```python
from build123d import *

# Parameters (mm, degrees)
MODEL_R                 = 1.5
SALIENTE_EXTRUIR1_DEPTH = 3


with BuildPart() as part:
    # Model → Saliente-Extruir1 (new body)
    with BuildSketch(Plane.XY):
        with BuildLine():
            Line((256.429131311, 228.742243614), (364.429131311, 228.742243614))
            ThreePointArc((364.429131311, 228.742243614), (367.611111826, 227.424224129), (368.929131311, 224.242243614))
            Line((368.929131311, 224.242243614), (368.929131311, 215.242243614))
            ThreePointArc((368.929131311, 215.242243614), (367.611111826, 212.060263099), (364.429131311, 210.742243614))
            Line((364.429131311, 210.742243614), (256.429131311, 210.742243614))
            ThreePointArc((256.429131311, 210.742243614), (253.247150795, 212.060263099), (251.929131311, 215.242243614))
            Line((251.929131311, 215.242243614), (251.929131311, 224.242243614))
            ThreePointArc((251.929131311, 224.242243614), (253.247150795, 227.424224129), (256.429131311, 228.742243614))
        make_face()
        with Locations((337.429131311, 215.242243614)):
            Circle(MODEL_R, mode=Mode.SUBTRACT)
        with Locations((319.429131311, 215.242243614)):
            Circle(MODEL_R, mode=Mode.SUBTRACT)
        with Locations((328.429131311, 215.242243614)):
            Circle(MODEL_R, mode=Mode.SUBTRACT)
        with Locations((310.429131311, 215.242243614)):
            Circle(MODEL_R, mode=Mode.SUBTRACT)
        with Locations((292.429131311, 215.242243614)):
            Circle(MODEL_R, mode=Mode.SUBTRACT)
        with Locations((301.429131311, 215.242243614)):
            Circle(MODEL_R, mode=Mode.SUBTRACT)
        with Locations((274.429131311, 215.242243614)):
            Circle(MODEL_R, mode=Mode.SUBTRACT)
        with Locations((283.429131311, 215.242243614)):
            Circle(MODEL_R, mode=Mode.SUBTRACT)
        with Locations((265.429131311, 215.242243614)):
            Circle(MODEL_R, mode=Mode.SUBTRACT)
        with Locations((256.429131311, 215.242243614)):
            Circle(MODEL_R, mode=Mode.SUBTRACT)
        with Locations((346.429131311, 215.242243614)):
            Circle(MODEL_R, mode=Mode.SUBTRACT)
        with Locations((355.429131311, 215.242243614)):
            Circle(MODEL_R, mode=Mode.SUBTRACT)
        with Locations((364.429131311, 215.242243614)):
            Circle(MODEL_R, mode=Mode.SUBTRACT)
        with BuildLine():
            Line((267.929131311, 222.617243614), (262.929131311, 222.617243614))
            ThreePointArc((262.929131311, 222.617243614), (262.398801225, 222.836913528), (262.179131311, 223.367243614))
            Line((262.179131311, 223.367243614), (262.179131311, 225.117243614))
            ThreePointArc((262.179131311, 225.117243614), (262.398801225, 225.6475737), (262.929131311, 225.867243614))
            Line((262.929131311, 225.867243614), (267.929131311, 225.867243614))
            ThreePointArc((267.929131311, 225.867243614), (268.459461397, 225.6475737), (268.679131311, 225.117243614))
            Line((268.679131311, 225.117243614), (268.679131311, 223.367243614))
            ThreePointArc((268.679131311, 223.367243614), (268.459461397, 222.836913528), (267.929131311, 222.617243614))
        make_face(mode=Mode.SUBTRACT)
        with BuildLine():
            Line((285.929131311, 222.617243614), (280.929131311, 222.617243614))
            ThreePointArc((280.929131311, 222.617243614), (280.398801225, 222.836913528), (280.179131311, 223.367243614))
            Line((280.179131311, 223.367243614), (280.179131311, 225.117243614))
            ThreePointArc((280.179131311, 225.117243614), (280.398801225, 225.6475737), (280.929131311, 225.867243614))
            Line((280.929131311, 225.867243614), (285.929131311, 225.867243614))
            ThreePointArc((285.929131311, 225.867243614), (286.459461397, 225.6475737), (286.679131311, 225.117243614))
            Line((286.679131311, 225.117243614), (286.679131311, 223.367243614))
            ThreePointArc((286.679131311, 223.367243614), (286.459461397, 222.836913528), (285.929131311, 222.617243614))
        make_face(mode=Mode.SUBTRACT)
        with BuildLine():
            Line((258.929131311, 222.617243614), (253.929131311, 222.617243614))
            ThreePointArc((253.929131311, 222.617243614), (253.398801225, 222.836913528), (253.179131311, 223.367243614))
            Line((253.179131311, 223.367243614), (253.179131311, 225.117243614))
            ThreePointArc((253.179131311, 225.117243614), (253.398801225, 225.6475737), (253.929131311, 225.867243614))
            Line((253.929131311, 225.867243614), (258.929131311, 225.867243614))
            ThreePointArc((258.929131311, 225.867243614), (259.459461397, 225.6475737), (259.679131311, 225.117243614))
            Line((259.679131311, 225.117243614), (259.679131311, 223.367243614))
            ThreePointArc((259.679131311, 223.367243614), (259.459461397, 222.836913528), (258.929131311, 222.617243614))
        make_face(mode=Mode.SUBTRACT)
        with BuildLine():
            Line((276.929131311, 222.617243614), (271.929131311, 222.617243614))
            ThreePointArc((271.929131311, 222.617243614), (271.398801225, 222.836913528), (271.179131311, 223.367243614))
            Line((271.179131311, 223.367243614), (271.179131311, 225.117243614))
            ThreePointArc((271.179131311, 225.117243614), (271.398801225, 225.6475737), (271.929131311, 225.867243614))
            Line((271.929131311, 225.867243614), (276.929131311, 225.867243614))
            ThreePointArc((276.929131311, 225.867243614), (277.459461397, 225.6475737), (277.679131311, 225.117243614))
            Line((277.679131311, 225.117243614), (277.679131311, 223.367243614))
            ThreePointArc((277.679131311, 223.367243614), (277.459461397, 222.836913528), (276.929131311, 222.617243614))
        make_face(mode=Mode.SUBTRACT)
        with BuildLine():
            Line((294.929131311, 222.617243614), (289.929131311, 222.617243614))
            ThreePointArc((289.929131311, 222.617243614), (289.398801225, 222.836913528), (289.179131311, 223.367243614))
            Line((289.179131311, 223.367243614), (289.179131311, 225.117243614))
            ThreePointArc((289.179131311, 225.117243614), (289.398801225, 225.6475737), (289.929131311, 225.867243614))
            Line((289.929131311, 225.867243614), (294.929131311, 225.867243614))
            ThreePointArc((294.929131311, 225.867243614), (295.459461397, 225.6475737), (295.679131311, 225.117243614))
            Line((295.679131311, 225.117243614), (295.679131311, 223.367243614))
            ThreePointArc((295.679131311, 223.367243614), (295.459461397, 222.836913528), (294.929131311, 222.617243614))
        make_face(mode=Mode.SUBTRACT)
        with BuildLine():
            Line((303.929131311, 222.617243614), (298.929131311, 222.617243614))
            ThreePointArc((298.929131311, 222.617243614), (298.398801225, 222.836913528), (298.179131311, 223.367243614))
            Line((298.179131311, 223.367243614), (298.179131311, 225.117243614))
            ThreePointArc((298.179131311, 225.117243614), (298.398801225, 225.6475737), (298.929131311, 225.867243614))
            Line((298.929131311, 225.867243614), (303.929131311, 225.867243614))
            ThreePointArc((303.929131311, 225.867243614), (304.459461397, 225.6475737), (304.679131311, 225.117243614))
            Line((304.679131311, 225.117243614), (304.679131311, 223.367243614))
            ThreePointArc((304.679131311, 223.367243614), (304.459461397, 222.836913528), (303.929131311, 222.617243614))
        make_face(mode=Mode.SUBTRACT)
        with BuildLine():
            Line((321.929131311, 222.617243614), (316.929131311, 222.617243614))
            ThreePointArc((316.929131311, 222.617243614), (316.398801225, 222.836913528), (316.179131311, 223.367243614))
            Line((316.179131311, 223.367243614), (316.179131311, 225.117243614))
            ThreePointArc((316.179131311, 225.117243614), (316.398801225, 225.6475737), (316.929131311, 225.867243614))
            Line((316.929131311, 225.867243614), (321.929131311, 225.867243614))
            ThreePointArc((321.929131311, 225.867243614), (322.459461397, 225.6475737), (322.679131311, 225.117243614))
            Line((322.679131311, 225.117243614), (322.679131311, 223.367243614))
            ThreePointArc((322.679131311, 223.367243614), (322.459461397, 222.836913528), (321.929131311, 222.617243614))
        make_face(mode=Mode.SUBTRACT)
        with BuildLine():
            Line((312.929131311, 222.617243614), (307.929131311, 222.617243614))
            ThreePointArc((307.929131311, 222.617243614), (307.398801225, 222.836913528), (307.179131311, 223.367243614))
            Line((307.179131311, 223.367243614), (307.179131311, 225.117243614))
            ThreePointArc((307.179131311, 225.117243614), (307.398801225, 225.6475737), (307.929131311, 225.867243614))
            Line((307.929131311, 225.867243614), (312.929131311, 225.867243614))
            ThreePointArc((312.929131311, 225.867243614), (313.459461397, 225.6475737), (313.679131311, 225.117243614))
            Line((313.679131311, 225.117243614), (313.679131311, 223.367243614))
            ThreePointArc((313.679131311, 223.367243614), (313.459461397, 222.836913528), (312.929131311, 222.617243614))
        make_face(mode=Mode.SUBTRACT)
        with BuildLine():
            Line((357.929131311, 222.617243614), (352.929131311, 222.617243614))
            ThreePointArc((352.929131311, 222.617243614), (352.398801225, 222.836913528), (352.179131311, 223.367243614))
            Line((352.179131311, 223.367243614), (352.179131311, 225.117243614))
            ThreePointArc((352.179131311, 225.117243614), (352.398801225, 225.6475737), (352.929131311, 225.867243614))
            Line((352.929131311, 225.867243614), (357.929131311, 225.867243614))
            ThreePointArc((357.929131311, 225.867243614), (358.459461397, 225.6475737), (358.679131311, 225.117243614))
            Line((358.679131311, 225.117243614), (358.679131311, 223.367243614))
            ThreePointArc((358.679131311, 223.367243614), (358.459461397, 222.836913528), (357.929131311, 222.617243614))
        make_face(mode=Mode.SUBTRACT)
        with BuildLine():
            Line((348.929131311, 222.617243614), (343.929131311, 222.617243614))
            ThreePointArc((343.929131311, 222.617243614), (343.398801225, 222.836913528), (343.179131311, 223.367243614))
            Line((343.179131311, 223.367243614), (343.179131311, 225.117243614))
            ThreePointArc((343.179131311, 225.117243614), (343.398801225, 225.6475737), (343.929131311, 225.867243614))
            Line((343.929131311, 225.867243614), (348.929131311, 225.867243614))
            ThreePointArc((348.929131311, 225.867243614), (349.459461397, 225.6475737), (349.679131311, 225.117243614))
            Line((349.679131311, 225.117243614), (349.679131311, 223.367243614))
            ThreePointArc((349.679131311, 223.367243614), (349.459461397, 222.836913528), (348.929131311, 222.617243614))
        make_face(mode=Mode.SUBTRACT)
        with BuildLine():
            Line((339.929131311, 222.617243614), (334.929131311, 222.617243614))
            ThreePointArc((334.929131311, 222.617243614), (334.398801225, 222.836913528), (334.179131311, 223.367243614))
            Line((334.179131311, 223.367243614), (334.179131311, 225.117243614))
            ThreePointArc((334.179131311, 225.117243614), (334.398801225, 225.6475737), (334.929131311, 225.867243614))
            Line((334.929131311, 225.867243614), (339.929131311, 225.867243614))
            ThreePointArc((339.929131311, 225.867243614), (340.459461397, 225.6475737), (340.679131311, 225.117243614))
            Line((340.679131311, 225.117243614), (340.679131311, 223.367243614))
            ThreePointArc((340.679131311, 223.367243614), (340.459461397, 222.836913528), (339.929131311, 222.617243614))
        make_face(mode=Mode.SUBTRACT)
        with BuildLine():
            Line((330.929131311, 222.617243614), (325.929131311, 222.617243614))
            ThreePointArc((325.929131311, 222.617243614), (325.398801225, 222.836913528), (325.179131311, 223.367243614))
            Line((325.179131311, 223.367243614), (325.179131311, 225.117243614))
            ThreePointArc((325.179131311, 225.117243614), (325.398801225, 225.6475737), (325.929131311, 225.867243614))
            Line((325.929131311, 225.867243614), (330.929131311, 225.867243614))
            ThreePointArc((330.929131311, 225.867243614), (331.459461397, 225.6475737), (331.679131311, 225.117243614))
            Line((331.679131311, 225.117243614), (331.679131311, 223.367243614))
            ThreePointArc((331.679131311, 223.367243614), (331.459461397, 222.836913528), (330.929131311, 222.617243614))
        make_face(mode=Mode.SUBTRACT)
        with BuildLine():
            Line((366.929131311, 222.617243614), (361.929131311, 222.617243614))
            ThreePointArc((361.929131311, 222.617243614), (361.398801225, 222.836913528), (361.179131311, 223.367243614))
            Line((361.179131311, 223.367243614), (361.179131311, 225.117243614))
            ThreePointArc((361.179131311, 225.117243614), (361.398801225, 225.6475737), (361.929131311, 225.867243614))
            Line((361.929131311, 225.867243614), (366.929131311, 225.867243614))
            ThreePointArc((366.929131311, 225.867243614), (367.459461397, 225.6475737), (367.679131311, 225.117243614))
            Line((367.679131311, 225.117243614), (367.679131311, 223.367243614))
            ThreePointArc((367.679131311, 223.367243614), (367.459461397, 222.836913528), (366.929131311, 222.617243614))
        make_face(mode=Mode.SUBTRACT)
    extrude(amount=SALIENTE_EXTRUIR1_DEPTH)


solid = part.part
```
Can you work these out from the model? Positions are in its coordinate system, mm. A direction names the side the tool comes from. Give positions to 0.01 mm unless a question says otherwise; leave off trailing zeros. Order: outer loops, then holes, each group sorted by start corner. A loop starts at its lowest first (then second) coordinate and runs counter-clockwise, first axis right, second up. Notation, with made-up numbers: (27, -19) - (80, -19) arc R26 ccw to (80, 19) - close; hole circle Ø3 at (5, -2). An arc over 180 degrees is marked (long way). Use a Markdown table: item, result. Add a question column.
Q1. If we mould it in two halves opening along X, with no side actions, what happens to faces 3 (the flat face through (310, 228.742, 1)), 4 (the cylindrical face through (253.28, 212.03, 1.48)), 5 (the cylindrical face through (254.93, 215.31, 1.48))? For each: released by +X, released by -X, zero draft, split by the parting line, or undercut.
Q2. Please list where these lines run through material, in increasing order: line 1 along Y through (x, z) = (290, 2); line 2 along Y through (x, z) = (257.5, 1.45); line 3 along Y through (x, z) = (329, 0.4).
Q3. On a 3-axis mill with a long thin cutter (end or side, diameter ignored), from which of +Z, -Z, +X, -X, +Y, -Y can I reach the whole of each face in a straight line? I mean faces 1 (the flat face through (283, 222.617, 1)), 2 (the flat face through (311, 220, 3)). Say none if no direction works.
Q4. If we section it at B-B on y = 227.25: Write out the boundary of the cut face in (x, z).
Q5. If we section it at A-A on z = 1.55: Count the separate pieces of the cut face and the enclosed holes in it, plus the area to 3 significant figures.
Answers follow:
| question | item | result |
|---|---|---|
| 1 | face 3 | zero draft |
| 1 | face 4 | released by -X |
| 1 | face 5 | undercut |
| 2 | line 1 | y = 210.74 to 222.62, 225.87 to 228.74 |
| 2 | line 2 | y = 210.74 to 214.19, 216.29 to 222.62, 225.87 to 228.74 |
| 2 | line 3 | y = 210.74 to 213.86, 216.63 to 222.62, 225.87 to 228.74 |
| 3 | face 1 | +Z, -Z |
| 3 | face 2 | +Z, +X, -X, +Y, -Y |
| 4 | outline | (253.08, 0) - (367.78, 0) - (367.78, 3) - (253.08, 3) - close |
| 5 | separate pieces | 1 |
| 5 | enclosed holes | 26 |
| 5 | area | 1,730 mm^2 |
